Model file for the job. Use its own axes, mm. A direction names the side the tool comes from. Round coordinates to 2 decimals unless told otherwise and drop trailing zeros. Order: outer loops, then holes, each group sorted by start corner. A loop starts at its lowest first (then second) coordinate and runs counter-clockwise, first axis right, second up. Notation, with made-up numbers: (20.5, -28.5) -> (32.5, -28.5) arc R24 ccw to (32.5, 7.5) -> close; hole circle Ø7 at (-16, 41.25). An arc over 180 degrees is marked (long way). Put each result on its own line as item: value. Start each with the question number.
Q1. 3-axis set-ups, long thin cutter, end or side, ignore diameter. For faces 4 (the face through (130, 6, -6.35)), 5 (the face through (56, 12, 25.4)), 6 (the face through (64, -6.35, 13)): which of +Z, -Z, +X, -X, +Y, -Y reach the whole face in a straight line?
Q2. Cut at B-B, the plane z = 18. List the corners of the cut face in (x, y).
Q3. Pull direction Y, two halves, no side cores. Call faces 1 (the face through (66.285, 18.866, 12.522)), 2 (the face through (31.75, -0.14, 12.52)), 3 (the face through (4, 19, -12.7)): released by +Y, released by -Y, zero draft, split by the parting line, or undercut.
Q4. Probe L1, parallel to Y at x = 64.5, z = 9; L2, parallel to Y at x = 127, z = -2; L3, parallel to X at y = -3.5, z = 21. List the from-to ranges inside material, lowest first.
Q5. Cut at A-A, the plane x = 0. List the corners of the cut face in (y, z), and give its area (3 significant figures).
Q6. Flat gauge pins, fed straight in: P1, Ø8, axis at x = 43, y = -11.5, coming from the -Z side; P2, Ø12, axis at y = -13.5, z = -1, coming from the -X side; P3, Ø7.5, axis at x = 127, y = 0, coming from the +Z side; P4, Ø7.5, axis at x = 131, y = 3, coming from the -Z side. Where does each tip first touch, or does it go through?
Q7. Cut at D-D, the plane y = 1.5. List the corners of the cut face in (x, z).
Q8. Cut at C-C, the plane y = 8.5. List the corners of the cut face in (x, z), and give its area (3 significant figures).
from build123d import *

# Parameters (mm, degrees)
F0_R     = 19.05
F0_R_2   = 6.35
F1_DEPTH = 25.4
F2_DEPTH = 6.35
F3_DEPTH = 12.7


with BuildPart() as f1:
    # F0 (on Top) → F1 (new body)
    with BuildSketch(Plane.XY):
        with BuildLine():
            ThreePointArc((2.54, -25.272681), (18.837144, -17.038838), (25.4, 0))
            ThreePointArc((25.4, 0), (18.837144, 17.038838), (2.54, 25.272681))
            ThreePointArc((2.54, 25.272681), (-25.4, 0), (2.54, -25.272681))
        make_face()
        Circle(F0_R, mode=Mode.SUBTRACT)
        with BuildLine():
            ThreePointArc((2.54, 25.272681), (18.837144, 17.038838), (25.4, 0))
            ThreePointArc((25.4, 0), (18.837144, -17.038838), (2.54, -25.272681))
            Line((2.54, -25.272681), (128.27, -12.63634))
            ThreePointArc((128.27, -12.63634), (114.3, 0), (128.27, 12.63634))
            Line((128.27, 12.63634), (2.54, 25.272681))
        make_face()
        with BuildLine():
            ThreePointArc((38.1, -6.35), (31.75, 0), (38.1, 6.35))
            Line((38.1, 6.35), (88.9, 6.35))
            ThreePointArc((88.9, 6.35), (95.25, 0), (88.9, -6.35))
            Line((88.9, -6.35), (38.1, -6.35))
        make_face(mode=Mode.SUBTRACT)
        with BuildLine():
            ThreePointArc((139.7, 0), (136.418572, 8.519419), (128.27, 12.63634))
            ThreePointArc((128.27, 12.63634), (114.3, 0), (128.27, -12.63634))
            ThreePointArc((128.27, -12.63634), (136.418572, -8.519419), (139.7, 0))
        make_face()
        with Locations((127, 0)):
            Circle(F0_R_2, mode=Mode.SUBTRACT)
    extrude(amount=F1_DEPTH)

    # F0 (on Top) → F2 (join)
    with BuildSketch(Plane.XY):
        with BuildLine():
            ThreePointArc((139.7, 0), (136.418572, 8.519419), (128.27, 12.63634))
            ThreePointArc((128.27, 12.63634), (114.3, 0), (128.27, -12.63634))
            ThreePointArc((128.27, -12.63634), (136.418572, -8.519419), (139.7, 0))
        make_face()
        with Locations((127, 0)):
            Circle(F0_R_2, mode=Mode.SUBTRACT)
    extrude(amount=-F2_DEPTH)

    # F0 (on Top) → F3 (join)
    with BuildSketch(Plane.XY):
        with BuildLine():
            ThreePointArc((2.54, -25.272681), (18.837144, -17.038838), (25.4, 0))
            ThreePointArc((25.4, 0), (18.837144, 17.038838), (2.54, 25.272681))
            ThreePointArc((2.54, 25.272681), (-25.4, 0), (2.54, -25.272681))
        make_face()
        Circle(F0_R, mode=Mode.SUBTRACT)
    extrude(amount=-F3_DEPTH)


solid = f1.part
Ans:
1. face 4: -Z, +X, +Y, -Y
1. face 5: +Z, +X, -X, +Y, -Y
1. face 6: +Z, -Z
2. outline: (2.54, -25.27) -> (128.27, -12.64) arc R12.7 ccw to (128.27, 12.64) -> (2.54, 25.27) arc R25.4 ccw (long way) to start; hole circle Ø38.1 at (0, 0); hole (38.1, -6.35) -> (88.9, -6.35) arc R6.35 ccw to (88.9, 6.35) -> (38.1, 6.35) arc R6.35 ccw to start; hole circle Ø12.7 at (127, 0)
3. face 1: released by +Y
3. face 2: undercut
3. face 3: zero draft
4. L1: y = -19.05 to -6.35, 6.35 to 19.05
4. L2: y = -12.7 to -6.35, 6.35 to 12.7
4. L3: x = -25.16 to -18.73, 18.73 to 32.8, 94.2 to 121.7, 132.3 to 139.21
5. outline: (-25.4, -12.7) -> (-19.05, -12.7) -> (-19.05, 25.4) -> (-25.4, 25.4) -> close; (19.05, -12.7) -> (25.4, -12.7) -> (25.4, 25.4) -> (19.05, 25.4) -> close
5. area: 484 mm^2
6. P1: stops at z = 0
6. P2: stops at x = -24.27
6. P3: passes through
6. P4: stops at z = -6.35
7. outline: (-25.36, -12.7) -> (-18.99, -12.7) -> (-18.99, 25.4) -> (-25.36, 25.4) -> close; (18.99, -12.7) -> (25.36, -12.7) -> (25.36, 0) -> (31.93, 0) -> (31.93, 25.4) -> (18.99, 25.4) -> close; (95.07, 0) -> (114.39, 0) -> (114.39, -6.35) -> (120.83, -6.35) -> (120.83, 25.4) -> (95.07, 25.4) -> close; (133.17, -6.35) -> (139.61, -6.35) -> (139.61, 25.4) -> (133.17, 25.4) -> close
8. outline: (-23.94, -12.7) -> (-17.05, -12.7) -> (-17.05, 25.4) -> (-23.94, 25.4) -> close; (17.05, -12.7) -> (23.94, -12.7) -> (23.94, 0) -> (117.56, 0) -> (117.56, -6.35) -> (136.44, -6.35) -> (136.44, 25.4) -> (17.05, 25.4) -> close
8. area: 3,500 mm^2
